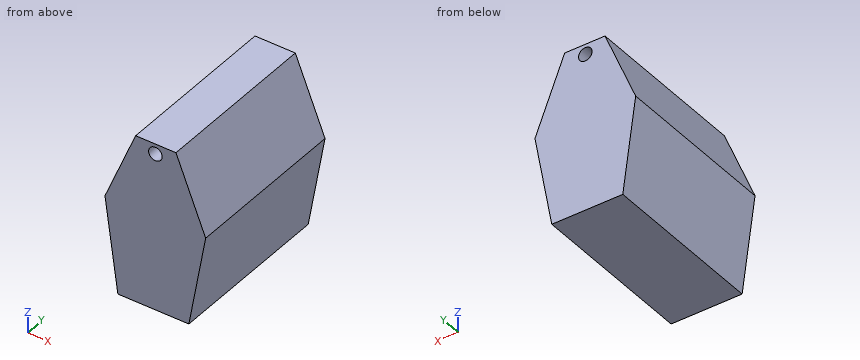
```python
from build123d import *

# Parameters (mm, degrees)
F0_R     = 10.0754230866
F1_DEPTH = 250


with BuildPart() as f1:
    # F0 (on Front) → F1 (new body)
    with BuildSketch(Plane.XZ):
        Polygon((1.384e-07, 130.2908220107), (-29.3460638914, 130.2908220107), (-75, 20.2908220107), (-55.803976953, -119.7091779893), (49.8614832759, -119.7091779893), (74.8796984553, 20.2908220107), (30.6539361086, 130.2908220107), align=None)
        with BuildLine():
            ThreePointArc((15, 115.2908220107), (-10.6066017667, 104.6842203418), (1.384e-07, 130.2908220107))
            ThreePointArc((1.384e-07, 130.2908220107), (10.6066017667, 125.8974236795), (15, 115.2908220107))
        make_face(mode=Mode.SUBTRACT)
        with BuildLine():
            ThreePointArc((15, 115.2908220107), (10.6066017667, 125.8974236795), (1.384e-07, 130.2908220107))
            ThreePointArc((1.384e-07, 130.2908220107), (-10.6066017667, 104.6842203418), (15, 115.2908220107))
        make_face()
        with Locations((0, 115.2908220107)):
            Circle(F0_R, mode=Mode.SUBTRACT)
    extrude(amount=F1_DEPTH)


solid = f1.part
```
Source: CAD feature listing. Evaluate the final solid. Frame: model axes, mm. Round coordinates to 2 decimals unless told otherwise and drop trailing zeros. Loops run counter-clockwise (first coordinate to the right, second up) from the corner with the lowest first, then second, coordinate; pieces in that order, holes last. Notation, with made-up numbers: M -4,-29 L 44,-29 A21 cw 44,-12 Z; hole C 49,-14.75 d3. An arc over 180 degrees is marked long. Put each result on its own line as item: value.
(1) First-contact query: pin 1 (10 mm diameter, centred on y = -202, z = -69, fed in from -X); pin 2 (18 mm diameter, centred on x = 0, z = 115.29, fed in from -Y); pin 3 (1.5 mm diameter, centred on x = 34, y = -167, fed in from +Z). Flat tips, straight axial feed; report the tip coordinate or a pass-through.
Solutions:
pin 1: x = -63.44
pin 2: through
pin 3: z = 123.83
(2) Section C-C, the plane z = -43. Return loops of the section in (x, y).
Solutions:
outline: M -66.32,-250 L 63.57,-250 L 63.57,0 L -66.32,0 Z
(3) Section D-D, the plane x = 38.5. Return loops of the section in (y, z).
Solutions:
outline: M -250,-119.71 L 0,-119.71 L 0,110.78 L -250,110.78 Z
(4) Ray query, line 1 (Z direction, x = 0, y = -64); line 2 (X direction, y = -152, z = 53); line 3 (X direction, y = -107.5, z = 111). Return the intervals inside material, ascending. Write a range as [from, to].
Solutions:
line 1: [-119.71, 105.22], [125.37, 130.29]
line 2: [-61.42, 61.73]
line 3: [-37.35, -9.12], [9.12, 38.41]
(5) Section B-B, the plane y = -182. Return loops of the section in (x, z).
Solutions:
outline: M -75,20.29 L -55.8,-119.71 L 49.86,-119.71 L 74.88,20.29 L 30.65,130.29 L -29.35,130.29 Z; hole C 0,115.29 d20.15
(6) Section A-A, the plane x = 0. Return loops of the section in (y, z), and give its area (3 significant figures).
Solutions:
outline: M -250,-119.71 L 0,-119.71 L 0,105.22 L -250,105.22 Z; M -250,125.37 L 0,125.37 L 0,130.29 L -250,130.29 Z
area: 57,500 mm²
